from build123d import *

# Parameters (mm, degrees)
SKETCH_R   = 21
SKETCH_R_2 = 22
PAD_DEPTH  = 30


with BuildPart() as part:
    # Sketch → Pad (new body)
    with BuildSketch(Plane.XY):
        with BuildLine():
            Line((-58.357879, -60.063078), (64.645731, -60.063078))
            ThreePointArc((64.645731, -60.063078), (77.632902, -54.683615), (83.012364, -41.696445))
            Line((83.012364, -41.696445), (83.012364, 80.611165))
            ThreePointArc((83.012364, 80.611165), (77.351981, 94.276539), (63.686607, 99.936922))
            Line((63.686607, 99.936922), (-57.470352, 99.936922))
            ThreePointArc((-57.470352, 99.936922), (-71.271156, 94.220442), (-76.987636, 80.419638))
            Line((-76.987636, 80.419638), (-76.987636, -41.433321))
            ThreePointArc((-76.987636, -41.433321), (-71.531106, -54.606548), (-58.357879, -60.063078))
        make_face()
        with Locations((-49.557964, -30.704547)):
            Circle(SKETCH_R, mode=Mode.SUBTRACT)
        with Locations((49.891115, 69.894362)):
            Circle(SKETCH_R, mode=Mode.SUBTRACT)
        with Locations((0.465053, 19.662022)):
            Circle(SKETCH_R_2, mode=Mode.SUBTRACT)
    extrude(amount=PAD_DEPTH)


solid = part.part
Can you work these out from the model? Positions are in its coordinate system, mm. Give positions to 0.01 mm unless a question says otherwise; leave off trailing zeros. Write each loop counter-clockwise with the first axis right and the second up, starting at its lowest first coordinate (ties: lowest second). Pieces come first, ordered by that corner, then holes. Notation, with made-up numbers: M -24.5,18 L 28.5,18 A22 ccw 28.5,53 Z; hole C 4,46.25 d3. An arc over 180 degrees is marked long. Answer in a Markdown table with one row per item. Add a question column.
Item 1: We'd pull the mould along X, two halves only. Please class faces 1 (the flat face through (83.012, 19, 15)), 2 (the cylindrical face through (-30.16, -38.75, 14.79)), 3 (the flat face through (4, 99.937, 15)): released by +X, released by -X, zero draft, split by the parting line, or undercut.
Item 2: Please list where these lines run through material, in increasing order: L1, parallel to X at y = 21, z = 15.5; L2, parallel to Y at x = 50.5, z = 25.5; L3, parallel to Y at x = 12.5, z = 2.25.
Item 3: Imagine slicing it at B-B, the plane x = -4. Write out the boundary of the cut face in (y, z).
Item 4: Imagine slicing it at C-C, the plane z = 10.25. Write out the boundary of the cut face in (x, y), plus the area to 3 significant figures.
Item 5: Imagine slicing it at A-A, the plane y = 5. Write out the boundary of the cut face in (x, z).
Evaluation:
| question | item | result |
|---|---|---|
| 1 | face 1 | released by +X |
| 1 | face 2 | undercut |
| 1 | face 3 | zero draft |
| 2 | L1 | x = -76.99 to -21.49, 22.42 to 83.01 |
| 2 | L2 | y = -60.06 to 48.9, 90.89 to 99.94 |
| 2 | L3 | y = -60.06 to 1.25, 38.08 to 99.94 |
| 3 | outline | M -60.06,0 L -1.88,0 L -1.88,30 L -60.06,30 Z; M 41.2,0 L 99.94,0 L 99.94,30 L 41.2,30 Z |
| 4 | outline | M -76.99,-41.43 A18.63 ccw -58.36,-60.06 L 64.65,-60.06 A18.37 ccw 83.01,-41.7 L 83.01,80.61 A19.33 ccw 63.69,99.94 L -57.47,99.94 A19.52 ccw -76.99,80.42 Z; hole C -49.56,-30.7 d42; hole C 0.47,19.66 d44; hole C 49.89,69.89 d42 |
| 4 | area | 21,000 mm² |
| 5 | outline | M -76.99,0 L -15.94,0 L -15.94,30 L -76.99,30 Z; M 16.87,0 L 83.01,0 L 83.01,30 L 16.87,30 Z |
